```python
from build123d import *

# Parameters (mm, degrees)
F1_R            = 8
F2_DEPTH        = 20
F4_DEPTH        = 4
F5_R            = 2
F6_DEPTH        = 9
F9_DEPTH        = 3.5
F10_W           = 7.2
F10_H           = 3.5
F11_DEPTH       = 9
F12_SIZE        = 1
F13_R           = 2.7
F14_DEPTH       = 13
F17_D           = 3.9
F17_DEPTH       = 9
F17_CBORE_D     = 7
F17_CBORE_DEPTH = 1
F17_TIP         = 1.1716782071


with BuildPart() as f2:
    # F1 (on Top) → F2 (new body)
    with BuildSketch(Plane.XY):
        Circle(F1_R)
    extrude(amount=F2_DEPTH)

    # F3 (on face) → F4 (join)
    with BuildSketch(Plane(origin=(0, 0, 0), x_dir=(1, 0, 0), z_dir=(0, 0, -1))):
        Polygon((-6, 3.4641016151), (-6, -3.4641016151), (0, -6.9282032303), (6, -3.4641016151), (6, 3.4641016151), (0, 6.9282032303), align=None)
    extrude(amount=F4_DEPTH)

    # F5 (on face) → F6 (cut)
    with BuildSketch(Plane(origin=(0, 0, -4), x_dir=(1, 0, 0), z_dir=(0, 0, -1))):
        Circle(F5_R)
    extrude(amount=-F6_DEPTH, mode=Mode.SUBTRACT)

    # F8 (on offset) → F9 (cut)
    with BuildSketch(Plane(origin=(0, 0, -2), x_dir=(1, 0, 0), z_dir=(0, 0, -1))):
        Polygon((3.6, -2.0784609691), (3.6, 2.0784609691), (0, 4.1569219382), (-3.6, 2.0784609691), (-3.6, -2.0784609691), (0, -4.1569219382), align=None)
    extrude(amount=-F9_DEPTH, mode=Mode.SUBTRACT)

    # F10 (on Front) → F11 (cut)
    with BuildSketch(Plane.XZ):
        with Locations((0, -0.25)):
            Rectangle(F10_W, F10_H)
    extrude(amount=F11_DEPTH, mode=Mode.SUBTRACT)

    # F12
    f12_edges = [f2.edges().sort_by_distance(p)[0] for p in [
        (-8, 0, 20),
    ]]
    chamfer(f12_edges, length=F12_SIZE)

    # F13 (on face) → F14 (cut)
    with BuildSketch(Plane.XY.offset(20)):
        Circle(F13_R)
    extrude(amount=-F14_DEPTH, mode=Mode.SUBTRACT)

    # F17
    with Locations(Plane.XZ.offset(8)):
        with Locations((0, 15)):
            CounterBoreHole(F17_D / 2, F17_CBORE_D / 2, F17_CBORE_DEPTH, depth=F17_DEPTH)
            with Locations((0, 0, -(F17_DEPTH + F17_TIP / 2))):  # 118° drill point
                Cone(0, F17_D / 2, F17_TIP, mode=Mode.SUBTRACT)


solid = f2.part
```
Geometry check sheet. Reference: the model listing, model coordinates, mm. A direction names the side the tool comes from. Coordinates: 2 decimals unless noted, no trailing zeros. Order: outer loops, then holes, each group sorted by start corner. A loop starts at its lowest first (then second) coordinate and runs counter-clockwise, first axis right, second up. Notation, with made-up numbers: (49.5, 46) - (93.5, 46) arc R24 ccw to (93.5, 77) - close; hole circle Ø3 at (-33.75, 48). An arc over 180 degrees is marked (long way). Answer as a JSON object with one key per item and string values. Group by question number.
Item 1: Sectioned sample at D-D, the plane z = 17.25. Record the cut outline in (x, y).
Item 2: Scan lines: probe 1 along Z at (x, y) = (0, -3.8); probe 2 along Z at (x, y) = (-2.75, -5.25); probe 3 along Z at (x, y) = (1.25, 2). Record each from-to range of solid material in increasing order.
Item 3: Sectioned sample at C-C, the plane y = -5.75. Give the number of separate pieces and of enclosed holes in the cut face, and give its area (3 significant figures).
Item 4: Depth check by flat-ended pin: pin 1 Ø3.5 at (x, y) = (0, 0) entering from -Z; pin 2 Ø5.5 at (x, z) = (1.5, 15.5) entering from -Y. Enter the tip coordinate at first touch or a pass-through.
Item 5: Draft check along X on faces 5 (the face through (3.709, -4.787, -2.416)), 6 (the face through (0, -3, 1.5)), 7 (the face through (-6, 0, -2)). Enter one of: +X half, -X half, draft (parallel to the pull), parting line (faces both ways), or undercut.
Item 6: Tool access check on faces 1 (the face through (0, 0, 7)), 2 (the face through (0, 2, 3)), 3 (the face through (-3.042, 5.172, -1.972)), 4 (the face through (3.6, -2, 0)). Record the directions out of +Z, -Z, +X, -X, +Y, -Y that give a thin tool (end or side, any length) a straight path to the whole face; none if there is none.
Item 7: Sectioned sample at A-A, the plane z = 0.5. Record the cut outline in (x, y), and give its area (3 significant figures).
Item 8: Sectioned sample at B-B, the plane y = 0. Record the cut outline in (x, z), and give its area (3 significant figures).
Resolved:
{
 "1": {"outline": "(-2.68, -7.54) - (-2.68, -7) - (2.68, -7) - (2.68, -7.54) arc R8 ccw (long way) to start; hole circle Ø5.4 at (0, 0)"},
 "2": {"probe 1": "-4 to -2, 1.5 to 13.05, 16.95 to 20", "probe 2": "-4 to -2, 1.5 to 20", "probe 3": "-4 to -2, 1.5 to 7"},
 "3": {"separate pieces": "2", "enclosed holes": "1", "area": "206 mm^2"},
 "4": {"pin 1": "z = 5", "pin 2": "y = -7.89"},
 "5": {"face 5": "+X half", "face 6": "undercut", "face 7": "-X half"},
 "6": {"face 1": "+Z", "face 2": "-Z", "face 3": "-Z, -X, +Y", "face 4": "-Y"},
 "7": {"outline": "(-3.6, -7.14) - (-3.6, 2.08) - (0, 4.16) - (3.6, 2.08) - (3.6, -7.14) arc R8 ccw (long way) to start", "area": "123 mm^2"},
 "8": {"outline": "(-8, 0) - (-6, 0) - (-6, -4) - (-2, -4) - (-2, -2) - (-3.6, -2) - (-3.6, 1.5) - (-2, 1.5) - (-2, 5) - (2, 5) - (2, 1.5) - (3.6, 1.5) - (3.6, -2) - (2, -2) - (2, -4) - (6, -4) - (6, 0) - (8, 0) - (8, 19) - (7, 20) - (2.7, 20) - (2.7, 7) - (-2.7, 7) - (-2.7, 20) - (-7, 20) - (-8, 19) - close", "area": "250 mm^2"}
}
